Read the model definition and answer for the solid it produces. Units are mm, in the model's axes. A direction names the side the tool comes from. Coordinates: 2 decimals unless noted, no trailing zeros. Order: outer loops, then holes, each group sorted by start corner. A loop starts at its lowest first (then second) coordinate and runs counter-clockwise, first axis right, second up.
```python
from build123d import *

# Parameters (mm, degrees)
SKETCH1_R           = 25
BOSS_EXTRUDE1_DEPTH = 70
BOSS_EXTRUDE2_DEPTH = 5
SKETCH3_R           = 125
BOSS_EXTRUDE3_DEPTH = 10


with BuildPart() as part:
    # Sketch1 → Boss-Extrude1 (new body)
    with BuildSketch(Plane(origin=(0, 0, 0), x_dir=(1, 0, 0), z_dir=(0, 1, 0))):
        with Locations(Location((0, 0, 0), (0, 0, 270))):
            Circle(SKETCH1_R)
    extrude(amount=BOSS_EXTRUDE1_DEPTH)

    # Sketch2 → Boss-Extrude2 (add)
    with BuildSketch(Plane(origin=(0, 40, 0), x_dir=(1, 0, 0), z_dir=(0, 1, 0))):
        with BuildLine():
            ThreePointArc((-49.768073149, -4.810290534), (49.989018115, 1.047887371), (-49.925935592, 2.720469675))
            ThreePointArc((-49.925935592, 2.720469675), (-99.550770715, -2.086818253), (-49.768073149, -4.810290534))
        make_face()
    extrude(amount=BOSS_EXTRUDE2_DEPTH)

    # Sketch3 → Boss-Extrude3 (add)
    with BuildSketch(Plane(origin=(0, 70, 0), x_dir=(1, 0, 0), z_dir=(0, 1, 0))):
        with Locations(Location((0, 0, 0), (0, 0, 270))):
            Circle(SKETCH3_R)
    extrude(amount=BOSS_EXTRUDE3_DEPTH)


solid = part.part
```
1) A cutting plane is placed at B-B, the plane z = -39.5. Determine the outline of the cut face in (x, y).
A:
outline: (-118.59, 70) - (118.59, 70) - (118.59, 80) - (-118.59, 80) - close; (-30.66, 40) - (30.66, 40) - (30.66, 45) - (-30.66, 45) - close
2) Straight lines are drawn through the part: line 1 (Y direction, x = -40, z = 10.5); line 2 (Y direction, x = 49, z = 106.5); line 3 (X direction, y = 57, z = -22). For each, find the intervals that lie inside material, in ascending order.
A:
line 1: y = 40 to 45, 70 to 80
line 2: y = 70 to 80
line 3: x = -11.87 to 11.87
3) A cutting plane is placed at C-C, the plane x = 14.5. Determine the outline of the cut face in (y, z), and give its area (3 significant figures).
A:
outline: (0, -20.37) - (40, -20.37) - (40, -47.85) - (45, -47.85) - (45, -20.37) - (70, -20.37) - (70, -124.16) - (80, -124.16) - (80, 124.16) - (70, 124.16) - (70, 20.37) - (45, 20.37) - (45, 47.85) - (40, 47.85) - (40, 20.37) - (0, 20.37) - close
area: 5,610 mm2
4) A cutting plane is placed at D-D, the plane y = 58.5. Determine the outline of the cut face in (x, z), and give its area (3 significant figures).
A:
outline: circle Ø50 at (0, 0)
area: 1,960 mm2
5) Determine the mould class of faces 1 (the flat face through (0, 0, 0)), 2 (the flat face through (2, 80, -2)), 3 (the flat face through (-26, 45, -1)) for opening direction Y: pulls with the +Y half, pulls with the -Y half, needs draft (parallel to the pull), parting line crosses it, or undercut.
A:
face 1: pulls with the -Y half
face 2: pulls with the +Y half
face 3: undercut
6) Flat-ended cylindrical pins translate along their axes: pin 1 Ø10 at (y, z) = (33, 9.5) entering from +X; pin 2 Ø1 at (x, z) = (-46, 99) entering from -Y; pin 3 Ø6 at (x, y) = (-8.5, 39) entering from -Z. Find the tip coordinate at first contact, or state that the pin passes through.
A:
pin 1: stops at x = 24.59
pin 2: stops at y = 70
pin 3: stops at z = -49.68
7) Which of the six approach directions +Z, -Z, +X, -X, +Y, -Y give full straight-line access (tool end or side, diameter ignored) to faces 4 (the cylindrical face through (7.509, 19.72, 23.846)), 5 (the cylindrical face through (7.509, 57.325, 23.846)), 6 (the cylindrical face through (5.5, 74.93, -124.88))?
A:
face 4: -Y
face 5: none
face 6: +Y, -Y
8) A cutting plane is placed at A-A, the plane x = -81. Determine the outline of the cut face in (y, z), and give its area (3 significant figures).
A:
outline: (40, -22.59) - (45, -22.59) - (45, 25.72) - (40, 25.72) - close; (70, -95.21) - (80, -95.21) - (80, 95.21) - (70, 95.21) - close
area: 2,150 mm2
